Verification items for this drawing (mm, ordinates from the low corner). A direction names the side the tool comes from. Coordinates: 2 decimals unless noted, no trailing zeros. Write each loop counter-clockwise with the first axis right and the second up, starting at its lowest first coordinate (ties: lowest second). Pieces come first, ordered by that corner, then holes. Notation, with made-up numbers: (4, -15.5) -> (59, -15.5) arc R37 ccw to (59, 22.5) -> close; hole circle Ø7 at (12.25, 41). An arc over 180 degrees is marked (long way). One line per item, written item: value. Start each with the question number.
1) Sectioned sample at B-B on y = 37. Enter the section's corners in (x, z) (1 decimal).
2) Sectioned sample at C-C on x = 38.5. Enter the section's corners in (y, z).
3) Set-up check for the marked faces 4 and 5: record each of +Z, -Z, +X, -X, +Y, -Y from which the full face is reachable in a straight line by a thin tool's end or side.
4) Sectioned sample at D-D on x = 25.5. Enter the section's corners in (y, z) (1 decimal), plus the area to 3 significant figures.
5) Sectioned sample at A-A on z = 21. Enter the section's corners in (x, y) (1 decimal).
6) Gauge pin test, flat ends, axial feed: P1, Ø5, axis at x = 35.5, y = 19.5, coming from the +Z side; P2, Ø12, axis at x = 29, y = 37.5, coming from the +Z side; P3, Ø6, axis at x = 21, y = 16, coming from the -Z side; P4, Ø3.5, axis at x = 21.17, y = 37, coming from the +Z side. Record the tip position at first contact, or that the pin passes through.
7) Scan lines: line 1 along X through (y, z) = (42, 12) (1 decimal); line 2 along X through (y, z) = (56.5, 45) (1 decimal); line 3 along Y through (x, z) = (26.5, 47.5). Record each from-to range of solid material in increasing order. Write a range as [from, to].
8) Draft check along X on the marked faces 1, 2 and 3. Enter one of: +X half, -X half, draft (parallel to the pull), parting line (faces both ways), or undercut.
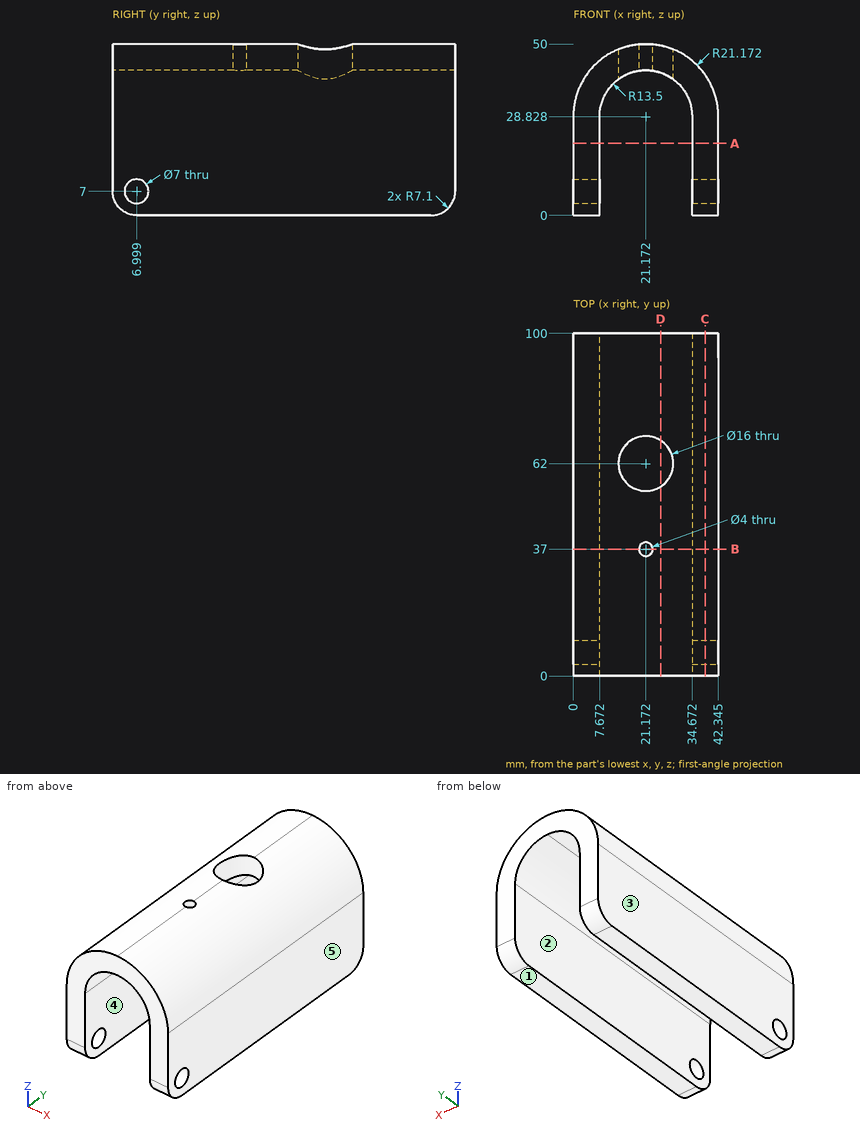
Answers:
1. outline: (0, 0) -> (7.7, 0) -> (7.7, 28.8) arc R13.5 cw to (19.2, 42.2) -> (19.2, 49.9) arc R21.2 ccw to (0, 28.8) -> close; (23.2, 42.2) arc R13.5 cw to (34.7, 28.8) -> (34.7, 0) -> (42.3, 0) -> (42.3, 28.8) arc R21.2 ccw to (23.2, 49.9) -> close
2. outline: (0, 7.1) arc R7.1 ccw to (7.1, 0) -> (92.9, 0) arc R7.1 ccw to (100, 7.1) -> (100, 40.99) -> (0, 40.99) -> close; hole circle Ø7 at (7, 7)
3. face 4: -Z, +Y, -Y
3. face 5: +Z, -Z, +X, +Y, -Y
4. outline: (0, 41.6) -> (55.3, 41.6) -> (55.3, 49.6) -> (0, 49.6) -> close; (68.7, 41.6) -> (100, 41.6) -> (100, 49.6) -> (68.7, 49.6) -> close
4. area: 687 mm2
5. outline: (0, 0) -> (7.7, 0) -> (7.7, 100) -> (0, 100) -> close; (34.7, 0) -> (42.3, 0) -> (42.3, 100) -> (34.7, 100) -> close
6. P1: stops at z = 46.39
6. P2: stops at z = 49.92
6. P3: stops at z = 41.95
6. P4: passes through
7. line 1: x = [0, 7.7], [34.7, 42.3]
7. line 2: x = [7.5, 15.4], [27, 34.8]
7. line 3: y = [0, 56.03], [67.97, 100]
8. face 1: draft
8. face 2: undercut
8. face 3: -X half
